from build123d import *

# Parameters (mm, degrees)
BOSS_EXTRUDE1_START     = -25
BOSS_EXTRUDE1_DEPTH     = 50
CUT_EXTRUDE1_DEPTH      = 341.53226913
CUT_EXTRUDE1_DEPTH_BACK = 341.53226913
CUT_EXTRUDE2_DEPTH      = 341.286795308
CUT_EXTRUDE2_DEPTH_BACK = 341.286795308
SKETCH4_R               = 20
CUT_EXTRUDE3_DEPTH      = 341.286795308
CUT_EXTRUDE3_DEPTH_BACK = 341.286795308
SKETCH6_R               = 12.5


# Read off the part's stored shape, not the designer's step: Boss-Extrude1
with BuildPart() as part:
    # Boss-Extrude1 outline → Boss-Extrude1 (new body)
    with BuildSketch(Plane.XY.offset(BOSS_EXTRUDE1_START)):
        with BuildLine():
            Line((175, 0), (215.218833807, 40.218833807))
            ThreePointArc((215.218833807, 40.218833807), (226.057471223, 56.440000887), (229.863494748, 75.574172084))
            add(Edge.make_bspline(
                [(229.863494748, 75.574172084), (229.863497015, 220.574172084), (130.657195822, 208), (130.657198498, 108), (160, 250), (60, 250)],
                knots=[0, 0, 0, 0, 0, 0, 1, 1, 1, 1, 1, 1], degree=5))
            Line((60, 250), (-60, 250))
            add(Edge.make_bspline(
                [(-60, 250), (-160, 250), (-130.657198498, 108), (-130.657195822, 208), (-229.863497015, 220.574172084), (-229.863494748, 75.574172084)],
                knots=[0, 0, 0, 0, 0, 0, 1, 1, 1, 1, 1, 1], degree=5))
            ThreePointArc((-229.863494748, 75.574172084), (-226.057471223, 56.440000887), (-215.218833807, 40.218833807))
            Line((-215.218833807, 40.218833807), (-175, 0))
            Line((-175, 0), (175, 0))
        make_face()
    extrude(amount=BOSS_EXTRUDE1_DEPTH)

    # Sketch2 → Cut-Extrude1 (cut, two sides: drawn at the far end of the back side and taken through both)
    with BuildSketch(Plane(origin=(0, 0, 0), x_dir=(0, 0, -1), z_dir=(1, 0, 0)).offset(-CUT_EXTRUDE1_DEPTH_BACK)):
        Polygon((23.039732542, -10), (-12.506441807, 260), (35, 260), (35, -10), align=None)
        Polygon((-23.039732542, 260), (12.506441807, -10), (-35, -10), (-35, 260), align=None)
    extrude(amount=CUT_EXTRUDE1_DEPTH + CUT_EXTRUDE1_DEPTH_BACK, mode=Mode.SUBTRACT)

    # Sketch4 → Cut-Extrude2 (cut, two sides: drawn at the far end of the back side and taken through both)
    with BuildSketch(Plane(origin=(0, 2.811189919, -21.353107392), x_dir=(-1, 0, 0), z_dir=(0, 0.13052619222005532, -0.99144486137381)).offset(-CUT_EXTRUDE2_DEPTH_BACK)):
        with Locations(Location((0, 124.321792579, 0), (0, 0, 90))):
            Circle(SKETCH4_R)
    extrude(amount=CUT_EXTRUDE2_DEPTH + CUT_EXTRUDE2_DEPTH_BACK, mode=Mode.SUBTRACT)

    # Sketch6 → Cut-Extrude3 (cut, two sides: drawn at the far end of the back side and taken through both)
    with BuildSketch(Plane(origin=(0, 2.811189919, -21.353107392), x_dir=(-1, 0, 0), z_dir=(0, 0.13052619222005532, -0.99144486137381)).offset(-CUT_EXTRUDE3_DEPTH_BACK)):
        with Locations(Location((150, 97.164552434, 0), (0, 0, 90))):
            Circle(SKETCH6_R)
    extrude(amount=CUT_EXTRUDE3_DEPTH + CUT_EXTRUDE3_DEPTH_BACK, mode=Mode.SUBTRACT)


solid = part.part
Read the model definition and answer for the solid it produces. Units are mm, in the model's axes. Round coordinates to 2 decimals unless told otherwise and drop trailing zeros. Write each loop counter-clockwise with the first axis right and the second up, starting at its lowest first coordinate (ties: lowest second). Pieces come first, ordered by that corner, then holes.
Q1. The mould has two halves that part along X. Classify faces 1 (the face through (-226.16, 56.69, -8.94)), 2 (the face through (-137.606, 96.84, -3.634)), 3 (the face through (1, 250, 16)): released by +X, released by -X, zero draft, split by the parting line, or undercut.
Values:
face 1: released by -X
face 2: undercut
face 3: zero draft
Q2. Flat-ended cylindrical pins translate along their axes: P1, Ø6, axis at y = 129, z = 3.5, coming from the +X side; P2, Ø4, axis at x = -99, y = 168.5, coming from the -Z side; P3, Ø12, axis at x = -138, y = 145, coming from the +Z side. Find the tip coordinate at first contact, or state that the pin passes through.
Values:
P1: stops at x = 223.93
P2: stops at z = 0.2
P3: stops at z = 8.69
Q3. Find section C-C on y = 47. Determine the outline of the cut face in (x, z), and give its area (3 significant figures).
Values:
outline: (-220.89, -15.54) - (220.89, -15.54) - (220.89, -5) - (-220.89, -5) - close
area: 4,650 mm2
Q4. Straight lines are drawn through the part: line 1 (X direction, y = 126, z = 5); line 2 (X direction, y = 92, z = -5); line 3 (Z direction, x = -139, y = 11). For each, find the intervals that lie inside material, in ascending order.
Values:
line 1: x = -223.93 to -19.96, 19.96 to 223.93
line 2: x = -229.32 to -160.61, -139.39 to 229.32
line 3: z = -20.28 to -9.74
Q5. Find section B-B on x = 52.5. Determine the outline of the cut face in (y, z), and give its area (3 significant figures).
Values:
outline: (0, -21.72) - (250, 11.19) - (250, 21.72) - (0, -11.19) - close
area: 2,630 mm2
Q6. Find section A-A on x = -5.5. Determine the outline of the cut face in (y, z).
Values:
outline: (0, -21.72) - (107.01, -7.64) - (105.64, 2.72) - (0, -11.19) - close; (143.77, 7.74) - (145.13, -2.62) - (250, 11.19) - (250, 21.72) - close
